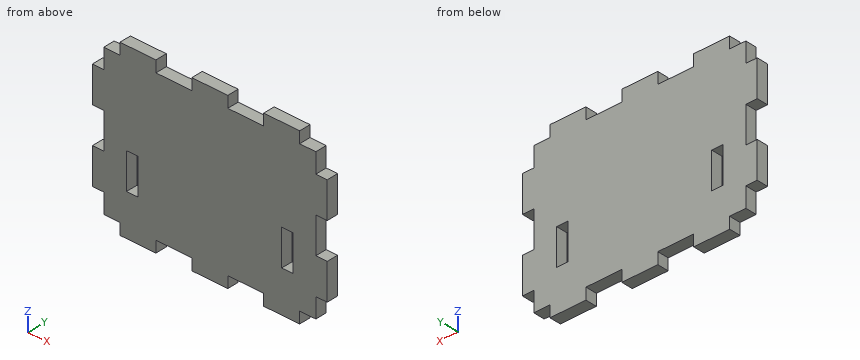
from build123d import *

# Parameters (mm, degrees)
SKETCH1_W           = 65.35
SKETCH1_H           = 47.35
BOSS_EXTRUDE1_DEPTH = 3.175
SKETCH2_W           = 4.5
SKETCH2_H           = 3.175
SKETCH2_W_2         = 3.175
SKETCH2_H_2         = 10
SKETCH2_W_3         = 10
CUT_EXTRUDE1_DEPTH  = 4.175
SKETCH3_W           = 3.175
SKETCH3_H           = 10
CUT_EXTRUDE2_DEPTH  = 4.175


with BuildPart() as part:
    # Sketch1 → Boss-Extrude1 (new body)
    with BuildSketch(Plane(origin=(0, 0, 0), x_dir=(1, 0, 0), z_dir=(0, 1, 0))):
        with Locations((32.675, 23.675)):
            Rectangle(SKETCH1_W, SKETCH1_H)
    extrude(amount=BOSS_EXTRUDE1_DEPTH)

    # Sketch2 → Cut-Extrude1 (cut, through all)
    with BuildSketch(Plane.XZ):
        with Locations((59.925, -45.7625)):
            Rectangle(SKETCH2_W, SKETCH2_H)
        Polygon((65.35, -38.675), (62.175, -38.675), (62.175, -44.175), (62.175, -47.35), (65.35, -47.35), align=None)
        with Locations((63.7625, -23.675)):
            Rectangle(SKETCH2_W_2, SKETCH2_H_2)
        Polygon((62.175, -8.675), (65.35, -8.675), (65.35, 0), (62.175, 0), (62.175, -3.175), align=None)
        with Locations((59.925, -1.5875)):
            Rectangle(SKETCH2_W, SKETCH2_H)
        with Locations((42.675, -1.5875)):
            Rectangle(SKETCH2_W_3, SKETCH2_H)
        with Locations((42.675, -45.7625)):
            Rectangle(SKETCH2_W_3, SKETCH2_H)
        with Locations((22.675, -45.7625)):
            Rectangle(SKETCH2_W_3, SKETCH2_H)
        with Locations((5.425, -45.7625)):
            Rectangle(SKETCH2_W, SKETCH2_H)
        Polygon((0, -47.35), (3.175, -47.35), (3.175, -44.175), (3.175, -38.675), (0, -38.675), align=None)
        with Locations((1.5875, -23.675)):
            Rectangle(SKETCH2_W_2, SKETCH2_H_2)
        Polygon((3.175, -3.175), (3.175, 0), (0, 0), (0, -8.675), (3.175, -8.675), align=None)
        with Locations((5.425, -1.5875)):
            Rectangle(SKETCH2_W, SKETCH2_H)
        with Locations((22.675, -1.5875)):
            Rectangle(SKETCH2_W_3, SKETCH2_H)
    extrude(amount=-CUT_EXTRUDE1_DEPTH, mode=Mode.SUBTRACT)

    # Sketch3 → Cut-Extrude2 (cut, through all)
    with BuildSketch(Plane.XZ):
        with Locations((54.2625, -30.791497658)):
            Rectangle(SKETCH3_W, SKETCH3_H)
        with Locations((11.0875, -30.791497658)):
            Rectangle(SKETCH3_W, SKETCH3_H)
    extrude(amount=-CUT_EXTRUDE2_DEPTH, mode=Mode.SUBTRACT)


solid = part.part
Check sheet for the modelled part. Datum: model origin and axes. Units: mm. Give positions to 0.01 mm unless a question says otherwise; leave off trailing zeros. Write each loop counter-clockwise with the first axis right and the second up, starting at its lowest first coordinate (ties: lowest second). Pieces come first, ordered by that corner, then holes. Notation, with made-up numbers: (-21.5, -14.75) -> (-3.5, -14.75) arc R19 ccw to (-3.5, 14.25) -> close; hole circle Ø7 at (88, -36). An arc over 180 degrees is marked (long way). Use one line per item in the form item = value. Start each with the question number.
1. Thickness scan on line 1 along X through (y, z) = (1.95, -3) (3 decimals); line 2 along X through (y, z) = (0.5, -34.5) (3 decimals); line 3 along Z through (x, y) = (11, 2). Record the ranges inside material, lowest first. Write a range as from..to.
2. Section check C-C (x = 43). Record the cut outline in (y, z) (3 decimals), and give its area (3 significant figures).
3. Section check A-A (y = 2.25). Count the separate pieces of the cut face and the enclosed holes in it, and give its area (3 significant figures).
4. Go/stop test with flat-tipped pins: P1, Ø1.5, axis at x = 58, z = -23, coming from the -Y side; P2, Ø1.6, axis at x = 5.5, y = 2, coming from the +Z side (3 decimals); P3, Ø1, axis at x = 2, y = 2.5, coming from the +Z side (3 decimals); P4, Ø1.6, axis at y = 1, z = -1.5, coming from the -X side (3 decimals). Record where each tip stops, or that it passes through.
5. Section check B-B (z = -7.5). Record the cut outline in (x, y) (3 decimals), and give its area (3 significant figures).
Conclusion:
q1.line_1 = 7.675..17.675, 27.675..37.675, 47.675..57.675
q1.line_2 = 0..9.5, 12.675..52.675, 55.85..65.35
q1.line_3 = -47.35..-35.79, -25.79..0
q2.outline = (0, -44.175) -> (3.175, -44.175) -> (3.175, -3.175) -> (0, -3.175) -> close
q2.area = 130 mm²
q3.separate_pieces = 1
q3.enclosed_holes = 2
q3.area = 2,670 mm²
q4.P1 = 0
q4.P2 = -3.175
q4.P3 = -8.675
q4.P4 = 7.675
q5.outline = (3.175, 0) -> (62.175, 0) -> (62.175, 3.175) -> (3.175, 3.175) -> close
q5.area = 187 mm²
